```python
from build123d import *

# Parameters (mm, degrees)
SKETCH1_W           = 110
SKETCH1_H           = 82
BOSS_EXTRUDE1_DEPTH = 5
SKETCH3_W           = 110
SKETCH3_H           = 2.5
BOSS_EXTRUDE2_DEPTH = 12.5
SKETCH4_W           = 2.5
SKETCH4_H           = 79.5
BOSS_EXTRUDE3_DEPTH = 12.5
SKETCH5_W           = 107.5
SKETCH5_H           = 2.5
BOSS_EXTRUDE4_DEPTH = 12.5
SKETCH6_W           = 2.5
SKETCH6_H           = 77
BOSS_EXTRUDE5_DEPTH = 12.5
SKETCH7_W           = 7
SKETCH7_H           = 10
CUT_EXTRUDE1_DEPTH  = 12.5
SKETCH8_W           = 12
SKETCH8_H           = 8
CUT_EXTRUDE2_DEPTH  = 2.54


with BuildPart() as part:
    # Sketch1 → Boss-Extrude1 (new body)
    with BuildSketch(Plane.XY):
        Rectangle(SKETCH1_W, SKETCH1_H)
    extrude(amount=BOSS_EXTRUDE1_DEPTH)

    # Sketch3 → Boss-Extrude2 (add)
    with BuildSketch(Plane.XY.offset(5)):
        with Locations((0, 39.75)):
            Rectangle(SKETCH3_W, SKETCH3_H)
    extrude(amount=BOSS_EXTRUDE2_DEPTH)

    # Sketch4 → Boss-Extrude3 (add)
    with BuildSketch(Plane.XY.offset(5)):
        with Locations((-53.75, -1.25)):
            Rectangle(SKETCH4_W, SKETCH4_H)
    extrude(amount=BOSS_EXTRUDE3_DEPTH)

    # Sketch5 → Boss-Extrude4 (add)
    with BuildSketch(Plane.XY.offset(5)):
        with Locations((1.25, -39.75)):
            Rectangle(SKETCH5_W, SKETCH5_H)
    extrude(amount=BOSS_EXTRUDE4_DEPTH)

    # Sketch6 → Boss-Extrude5 (add)
    with BuildSketch(Plane.XY.offset(5)):
        with Locations((53.75, 0)):
            Rectangle(SKETCH6_W, SKETCH6_H)
    extrude(amount=BOSS_EXTRUDE5_DEPTH)

    # Sketch7 → Cut-Extrude1 (cut)
    with BuildSketch(Plane.XY.offset(5)):
        with Locations((22, -20.7)):
            Rectangle(SKETCH7_W, SKETCH7_H)
    extrude(amount=-CUT_EXTRUDE1_DEPTH, mode=Mode.SUBTRACT)

    # Sketch8 → Cut-Extrude2 (cut)
    with BuildSketch(Plane.XZ.offset(41)):
        with Locations((12.06587737, 8.792437031)):
            Rectangle(SKETCH8_W, SKETCH8_H)
    extrude(amount=-CUT_EXTRUDE2_DEPTH, mode=Mode.SUBTRACT)


solid = part.part
```
Here's how the part is built. I have some questions about the finished solid (model axes, mm). A direction names the side the tool comes from. Coordinates: 2 decimals unless noted, no trailing zeros. Write each loop counter-clockwise with the first axis right and the second up, starting at its lowest first coordinate (ties: lowest second). Pieces come first, ordered by that corner, then holes. Notation, with made-up numbers: (-34, 54) - (-16, 54) arc R19 ccw to (-16, 72) - close; hole circle Ø10 at (43.25, 84.25). An arc over 180 degrees is marked (long way). One line per item, written item: value.
1) Suppose I cut it at C-C on y = 7.5. Write out the boundary of the cut face in (x, z).
Model answer:
outline: (-55, 0) - (55, 0) - (55, 17.5) - (52.5, 17.5) - (52.5, 5) - (-52.5, 5) - (-52.5, 17.5) - (-55, 17.5) - close
2) Suppose I cut it at D-D on x = 2. Write out the boundary of the cut face in (y, z), and give its area (4 significant figures).
Model answer:
outline: (-41, 0) - (41, 0) - (41, 17.5) - (38.5, 17.5) - (38.5, 5) - (-38.5, 5) - (-38.5, 17.5) - (-41, 17.5) - close
area: 472.5 mm²
3) Suppose I cut it at A-A on x = 22. Write out the boundary of the cut face in (y, z), and give its area (4 significant figures).
Model answer:
outline: (-41, 0) - (-25.7, 0) - (-25.7, 5) - (-38.5, 5) - (-38.5, 17.5) - (-41, 17.5) - close; (-15.7, 0) - (41, 0) - (41, 17.5) - (38.5, 17.5) - (38.5, 5) - (-15.7, 5) - close
area: 422.5 mm²
4) I need wall thicknesses on line 1 along X through (y, z) = (-18.5, 8.5); line 2 along Y through (x, z) = (40.5, 9); line 3 along Z through (x, y) = (40, -30.5). Which ranges of each line are inside material? Lowest first, please.
Model answer:
line 1: x = -55 to -52.5, 52.5 to 55
line 2: y = -41 to -38.5, 38.5 to 41
line 3: z = 0 to 5
5) Suppose I cut it at B-B on z = 9.25. Write out the boundary of the cut face in (x, y), and give its area (3 significant figures).
Model answer:
outline: (-55, -41) - (6.07, -41) - (6.07, -38.5) - (-52.5, -38.5) - (-52.5, 38.5) - (52.5, 38.5) - (52.5, -38.5) - (18.07, -38.5) - (18.07, -41) - (55, -41) - (55, 41) - (-55, 41) - close
area: 905 mm²
6) On a 3-axis mill with a long thin cutter (end or side, diameter ignored), from which of +Z, -Z, +X, -X, +Y, -Y can I reach the whole of each face in a straight line? I mean faces 1 (the flat face through (-1, 1, 5)), 2 (the flat face through (25.5, -21, 3)), 3 (the flat face through (-1, 1, 0)), 4 (the flat face through (12, -40, 12.792)), 5 (the flat face through (-4, -39, 17.5)). Say none if no direction works.
Model answer:
face 1: +Z
face 2: +Z, -Z
face 3: -Z, +X, -X, +Y, -Y
face 4: -Y
face 5: +Z, +X, -X, +Y, -Y
7) We'd pull the mould along Y, two halves only. Please class faces 6 (the flat face through (55, -1, 9)), 7 (the flat face through (-1, 41, 9)), 8 (the flat face through (-1, -41, 9)), 9 (the flat face through (22, -25.7, 3)): pulls with the +Y half, pulls with the -Y half, needs draft (parallel to the pull), parting line crosses it, or undercut.
Model answer:
face 6: needs draft
face 7: pulls with the +Y half
face 8: pulls with the -Y half
face 9: undercut
8) I'm going to push a flat-ended pin straight in: P1, Ø23, axis at x = 6.5, y = -15.5, coming from the +Z side. Where does the tip first touch, or does it pass through?
Model answer:
P1: stops at z = 5
